```python
from build123d import *

# Parameters (mm, degrees)
SKETCH_1_W          = 170
SKETCH_1_H          = 90
EXTRUDE_1_DEPTH     = 2
SKETCH_4_R          = 2.1
CUT_EXTRUDE_5_DEPTH = 10
FILLET_1_R          = 4
CUT_EXTRUDE_6_DEPTH = 112.748746927
SKETCH_7_R          = 1.6
CUT_EXTRUDE_7_DEPTH = 112.748746927
FILLET_2_R          = 4
FILLET_3_R          = 12


with BuildPart() as part:
    # 草图1 → 凸台-拉伸1 (new body)
    with BuildSketch(Plane.XY):
        with Locations((-10.625, 12.789634146)):
            Rectangle(SKETCH_1_W, SKETCH_1_H)
    extrude(amount=EXTRUDE_1_DEPTH)

    # 草图4 → 切除-拉伸5 (cut)
    with BuildSketch(Plane.XY.offset(2)):
        with Locations((59.375, -27.210365854)):
            Circle(SKETCH_4_R)
        with Locations((-80.625, -27.210365854)):
            Circle(SKETCH_4_R)
        with Locations((69.375, 47.789634146)):
            Circle(SKETCH_4_R)
        with Locations((-90.625, 47.789634146)):
            Circle(SKETCH_4_R)
    extrude(amount=-CUT_EXTRUDE_5_DEPTH, mode=Mode.SUBTRACT)

    # 圆角1
    fillet_1_edges = [part.edges().sort_by_distance(p)[0] for p in [
        (74.375, -32.210365854, 1),
        (-95.625, -32.210365854, 1),
    ]]
    fillet(fillet_1_edges, radius=FILLET_1_R)

    # 草图5 → 切除-拉伸6 (cut, through all)
    with BuildSketch(Plane.XY.offset(2)):
        Polygon((-73.625, 40.789634146), (52.375, 40.789634146), (52.375, 47.789634146), (52.375, 57.789634146), (2.375, 57.789634146), (-4.625, 57.789634146), (-73.625, 57.789634146), align=None)
    extrude(amount=-CUT_EXTRUDE_6_DEPTH, mode=Mode.SUBTRACT)

    # 草图7 → 切除-拉伸7 (cut, through all)
    with BuildSketch(Plane.XY.offset(2)):
        with Locations((49.375, 32.789634146)):
            Circle(SKETCH_7_R)
        with Locations((49.375, -17.210365854)):
            Circle(SKETCH_7_R)
        with Locations(Location((-70.625, -17.210365854, 0), (0, 0, 180))):
            Circle(SKETCH_7_R)
        with Locations(Location((-70.625, 32.789634146, 0), (0, 0, 180))):
            Circle(SKETCH_7_R)
    extrude(amount=-CUT_EXTRUDE_7_DEPTH, mode=Mode.SUBTRACT)

    # 圆角2
    fillet_2_edges = [part.edges().sort_by_distance(p)[0] for p in [
        (52.375, 40.789634146, 1),
        (-73.625, 40.789634146, 1),
        (-73.625, 57.789634146, 1),
        (52.375, 57.789634146, 1),
    ]]
    fillet(fillet_2_edges, radius=FILLET_2_R)

    # 圆角3
    fillet_3_edges = [part.edges().sort_by_distance(p)[0] for p in [
        (-95.625, 57.789634146, 1),
        (74.375, 57.789634146, 1),
    ]]
    fillet(fillet_3_edges, radius=FILLET_3_R)


solid = part.part
```
The model under review builds one solid part; all positions refer to its coordinate system, in mm. A direction names the side the tool comes from. Give positions to 0.01 mm unless a question says otherwise; leave off trailing zeros. Write each loop counter-clockwise with the first axis right and the second up, starting at its lowest first coordinate (ties: lowest second). Pieces come first, ordered by that corner, then holes. Notation, with made-up numbers: (-2, -10) -> (19, -10) arc R20 cw to (19, -6) -> close; hole circle Ø5 at (28.5, -37.5). An arc over 180 degrees is marked (long way). Answer in a Markdown table with one row per item.
1) Clearance check with flat-ended pins moving along their axes: P1, Ø1, axis at x = -31, z = 1.5, coming from the +Y side; P2, Ø1, axis at y = 50.5, z = 0.5, coming from the -X side. State where each tip first meets the part, or that it passes through.
Worked answers:
| item | result |
|---|---|
| P1 | y = 40.79 |
| P2 | x = -94.86 |
2) For L1, parallel to Y at x = 50, z = 0.35; L2, parallel to Y at x = 22, z = 1.8; L3, parallel to Y at x = -81, z = 0.3, list the stretches that pass through material, from the lowest coordinate up. Write a range as [from, to].
Worked answers:
| item | result |
|---|---|
| L1 | [-32.21, -18.68], [-15.74, 31.32], [34.26, 41.13] |
| L2 | [-32.21, 40.79] |
| L3 | [-32.21, -29.28], [-25.14, 57.79] |
3) Add section A-A on y = 52. State the section outline as (x, z) points (3 decimals), plus the area to 3 significant figures.
Worked answers:
| item | result |
|---|---|
| outline | (-93.893, 0) -> (-73.625, 0) -> (-73.625, 2) -> (-93.893, 2) -> close; (52.375, 0) -> (72.643, 0) -> (72.643, 2) -> (52.375, 2) -> close |
| area | 81.1 mm² |
4) Add section B-B on z = 1.7. Count the separate pieces of the cut face and the enclosed holes in it, plus the area to 3 significant figures.
Worked answers:
| item | result |
|---|---|
| separate pieces | 1 |
| enclosed holes | 8 |
| area | 13,000 mm² |
5) Mouldability with a two-part tool opening along X and no side actions: class faces 3 (the cylindrical face through (53.52, 56.59, 0.99)), 4 (the cylindrical face through (-92.016, 54.368, 1.014)), 5 (the cylindrical face through (73.17, -31.07, 1.01)) as +X half, -X half, draft (parallel to the pull), parting line (faces both ways), or undercut.
Worked answers:
| item | result |
|---|---|
| face 3 | undercut |
| face 4 | -X half |
| face 5 | +X half |
6) Tool access review of faces 1 (the cylindrical face through (-74.83, 56.65, 0.99)), 2 (the cylindrical face through (-82.723, -27.118, 1.014)): name each direction out of +Z, -Z, +X, -X, +Y, -Y from which nothing blocks a thin tool from reaching the whole face with its end or side.
Worked answers:
| item | result |
|---|---|
| face 1 | +Z, -Z, +Y |
| face 2 | +Z, -Z |
7) Add section C-C on x = -17.5. State the section outline as (y, z) points.
Worked answers:
| item | result |
|---|---|
| outline | (-32.21, 0) -> (40.79, 0) -> (40.79, 2) -> (-32.21, 2) -> close |
